from build123d import *

# Parameters (mm, degrees)
F0_W     = 70
F0_H     = 104
F1_DEPTH = 3
F2_R     = 5
F4_D     = 11
F6_DEPTH = 444
F9_DEPTH = 123
F10_D    = 11


with BuildPart() as f1:
    # F0 (on Front) → F1 (new body)
    with BuildSketch(Plane.XZ):
        with Locations((-71.837332, 40.87914)):
            Rectangle(F0_W, F0_H)
    extrude(amount=F1_DEPTH)

    # F2
    f2_edges = [f1.edges().sort_by_distance(p)[0] for p in [
        (-36.837332, -1.5, 92.87914),
        (-106.837332, -1.5, 92.87914),
        (-106.837332, -1.5, -11.12086),
        (-36.837332, -1.5, -11.12086),
    ]]
    fillet(f2_edges, radius=F2_R)

    # F4 (through all)
    with Locations(Plane.XZ.offset(3)):
        with Locations((-49.837332, 1.87914), (-93.837332, 1.87914), (-93.837332, 79.87914), (-49.837332, 79.87914)):
            Hole(F4_D / 2)

    # F5 (on face) → F6 (join)
    with BuildSketch(Plane.XZ.offset(3)):
        with BuildLine():
            ThreePointArc((-60.337332, 58.87914), (-60.923118, 60.293354), (-62.337332, 60.87914))
            Line((-62.337332, 60.87914), (-81.337332, 60.87914))
            ThreePointArc((-81.337332, 60.87914), (-82.751546, 60.293354), (-83.337332, 58.87914))
            Line((-83.337332, 58.87914), (-83.337332, 22.87914))
            ThreePointArc((-83.337332, 22.87914), (-82.751546, 21.464927), (-81.337332, 20.87914))
            Line((-81.337332, 20.87914), (-62.337332, 20.87914))
            ThreePointArc((-62.337332, 20.87914), (-60.923118, 21.464927), (-60.337332, 22.87914))
            Line((-60.337332, 22.87914), (-60.337332, 30.87914))
            Line((-60.337332, 30.87914), (-61.837332, 30.87914))
            Line((-61.837332, 30.87914), (-61.837332, 23.37914))
            ThreePointArc((-61.837332, 23.37914), (-62.130225, 22.672034), (-62.837332, 22.37914))
            Line((-62.837332, 22.37914), (-80.837332, 22.37914))
            ThreePointArc((-80.837332, 22.37914), (-81.544439, 22.672034), (-81.837332, 23.37914))
            Line((-81.837332, 23.37914), (-81.837332, 58.37914))
            ThreePointArc((-81.837332, 58.37914), (-81.544439, 59.086247), (-80.837332, 59.37914))
            Line((-80.837332, 59.37914), (-62.837332, 59.37914))
            ThreePointArc((-62.837332, 59.37914), (-62.130225, 59.086247), (-61.837332, 58.37914))
            Line((-61.837332, 58.37914), (-61.837332, 50.87914))
            Line((-61.837332, 50.87914), (-60.337332, 50.87914))
            Line((-60.337332, 50.87914), (-60.337332, 58.87914))
        make_face()
    extrude(amount=F6_DEPTH)

    # F7 (on face) → F9 (join)
    with BuildSketch(Plane.XZ.offset(447)):
        with BuildLine():
            ThreePointArc((-62.837332, 59.37914), (-62.130225, 59.086247), (-61.837332, 58.37914))
            Line((-61.837332, 58.37914), (-61.837332, 50.87914))
            Line((-61.837332, 50.87914), (-60.337332, 50.87914))
            Line((-60.337332, 50.87914), (-60.337332, 58.87914))
            ThreePointArc((-60.337332, 58.87914), (-60.923118, 60.293354), (-62.337332, 60.87914))
            Line((-62.337332, 60.87914), (-81.337332, 60.87914))
            ThreePointArc((-81.337332, 60.87914), (-82.751546, 60.293354), (-83.337332, 58.87914))
            Line((-83.337332, 58.87914), (-83.337332, 22.87914))
            ThreePointArc((-83.337332, 22.87914), (-82.751546, 21.464927), (-81.337332, 20.87914))
            Line((-81.337332, 20.87914), (-62.337332, 20.87914))
            ThreePointArc((-62.337332, 20.87914), (-60.923118, 21.464927), (-60.337332, 22.87914))
            Line((-60.337332, 22.87914), (-60.337332, 30.87914))
            Line((-60.337332, 30.87914), (-61.837332, 30.87914))
            Line((-61.837332, 30.87914), (-61.837332, 23.37914))
            ThreePointArc((-61.837332, 23.37914), (-62.130225, 22.672034), (-62.837332, 22.37914))
            Line((-62.837332, 22.37914), (-80.837332, 22.37914))
            ThreePointArc((-80.837332, 22.37914), (-81.544439, 22.672034), (-81.837332, 23.37914))
            Line((-81.837332, 23.37914), (-81.837332, 58.37914))
            ThreePointArc((-81.837332, 58.37914), (-81.544439, 59.086247), (-80.837332, 59.37914))
            Line((-80.837332, 59.37914), (-62.837332, 59.37914))
        make_face()
    extrude(amount=F9_DEPTH)

    # F10 (through all)
    with Locations(Plane(origin=(-83.337332, 0, 0), x_dir=(0, -1, 0), z_dir=(-1, 0, 0))):
        with Locations((544.8542, 40.87914)):
            Hole(F10_D / 2)


solid = f1.part
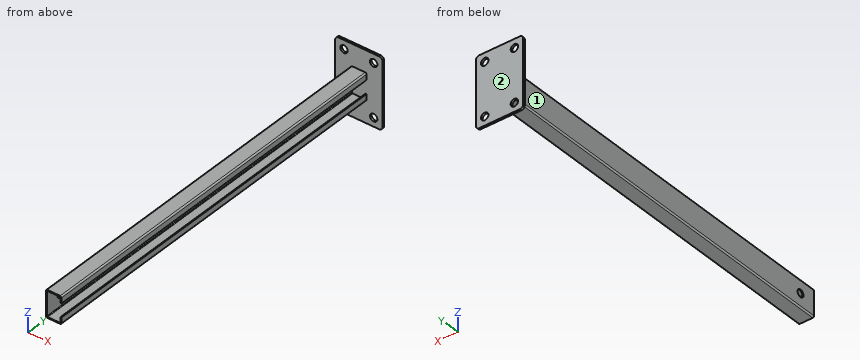
Could you check a few things on this model? Use its own coordinates, in mm. Face numbers are marked on the shaded views. A direction names the side the tool comes from. Give positions to 0.01 mm unless a question says otherwise; leave off trailing zeros. Order: outer loops, then holes, each group sorted by start corner. A loop starts at its lowest first (then second) coordinate and runs counter-clockwise, first axis right, second up. Notation, with made-up numbers: (57, 55) -> (96, 55) arc R15 ccw to (96, 72) -> close; hole circle Ø3 at (-8.75, 39.5). An arc over 180 degrees is marked (long way). Answer in a Markdown table with one row per item. Add a question column.
Item 1: I'm going to push flat-ended pins straight in: P1, Ø14.5, axis at x = -93.84, z = 79.88, coming from the -Y side; P2, Ø1.6, axis at x = -61, y = -360, coming from the -Z side; P3, Ø9, axis at x = -70, y = -210.5, coming from the -Z side. Where does each tip first touch, or does it pass through?
Item 2: Imagine slicing it at C-C (z = 12.5). List the corners of the cut face in (x, y) for me, and give its area (3 significant figures).
Item 3: Imagine slicing it at A-A (x = -93.5). List the corners of the cut face in (y, z) for me, and give its area (3 significant figures).
Item 4: Please list where these lines run through material, in increasing order: probe 1 along Z at (x, y) = (-62, -365); probe 2 along Z at (x, y) = (-79.5, -72.5); probe 3 along X at (y, z) = (-102, 56.5).
Item 5: Imagine slicing it at B-B (y = -151). List the corners of the cut face in (x, z) for me, and give its area (3 significant figures).
Item 6: For the marked faces 1 and 2, which set-ups out of +Z, -Z, +X, -X, +Y, -Y let a thin tool reach every point of the face, with its end or its side?
Result:
| question | item | result |
|---|---|---|
| 1 | P1 | y = -3 |
| 1 | P2 | z = 20.95 |
| 1 | P3 | z = 20.88 |
| 2 | outline | (-106.84, -3) -> (-36.84, -3) -> (-36.84, 0) -> (-106.84, 0) -> close |
| 2 | area | 210 mm2 |
| 3 | outline | (-3, -11.12) -> (0, -11.12) -> (0, -3.61) -> (-3, -3.61) -> close; (-3, 7.37) -> (0, 7.37) -> (0, 74.39) -> (-3, 74.39) -> close; (-3, 85.37) -> (0, 85.37) -> (0, 92.88) -> (-3, 92.88) -> close |
| 3 | area | 246 mm2 |
| 4 | probe 1 | 20.91 to 22.83, 58.93 to 60.85 |
| 4 | probe 2 | 20.88 to 22.38, 59.38 to 60.88 |
| 4 | probe 3 | -83.34 to -81.84, -61.84 to -60.34 |
| 5 | outline | (-83.34, 22.88) arc R2 ccw to (-81.34, 20.88) -> (-62.34, 20.88) arc R2 ccw to (-60.34, 22.88) -> (-60.34, 30.88) -> (-61.84, 30.88) -> (-61.84, 23.38) arc R1 cw to (-62.84, 22.38) -> (-80.84, 22.38) arc R1 cw to (-81.84, 23.38) -> (-81.84, 58.38) arc R1 cw to (-80.84, 59.38) -> (-62.84, 59.38) arc R1 cw to (-61.84, 58.38) -> (-61.84, 50.88) -> (-60.34, 50.88) -> (-60.34, 58.88) arc R2 ccw to (-62.34, 60.88) -> (-81.34, 60.88) arc R2 ccw to (-83.34, 58.88) -> close |
| 5 | area | 147 mm2 |
| 6 | face 1 | +Z, -Z, -X, -Y |
| 6 | face 2 | +Z, -Z, +X, -X, +Y |
